Input: part model. Units: mm. Frame: model coordinates. A direction names the side the tool comes from. Give positions to 0.01 mm unless a question says otherwise; leave off trailing zeros. Loops run counter-clockwise (first coordinate to the right, second up) from the corner with the lowest first, then second, coordinate; pieces in that order, holes last.
from build123d import *

# Parameters (mm, degrees)
SKETCH1_W                               = 80
SKETCH1_H                               = 80
SKETCH1_R                               = 2.55
SKETCH1_R_2                             = 2.05
BOSS_EXTRUDE1_DEPTH                     = 7
CBORE_FOR_5_64_EJECTOR_PIN1_D           = 1.984375
CBORE_FOR_5_64_EJECTOR_PIN1_CBORE_D     = 5.953125
CBORE_FOR_5_64_EJECTOR_PIN1_CBORE_DEPTH = 2.175


with BuildPart() as part:
    # Sketch1 → Boss-Extrude1 (new body)
    with BuildSketch(Plane(origin=(0, 0, 0), x_dir=(1, 0, 0), z_dir=(0, 1, 0))):
        with Locations((0, 18)):
            Rectangle(SKETCH1_W, SKETCH1_H)
        with Locations((-30, 15)):
            Circle(SKETCH1_R, mode=Mode.SUBTRACT)
        with Locations((30, 15)):
            Circle(SKETCH1_R, mode=Mode.SUBTRACT)
        with Locations((30, -15)):
            Circle(SKETCH1_R, mode=Mode.SUBTRACT)
        with Locations((-30, -15)):
            Circle(SKETCH1_R, mode=Mode.SUBTRACT)
        with Locations((-26.5, 53)):
            Circle(SKETCH1_R_2, mode=Mode.SUBTRACT)
        with Locations((26.5, 53)):
            Circle(SKETCH1_R_2, mode=Mode.SUBTRACT)
        with Locations((26.5, 33)):
            Circle(SKETCH1_R_2, mode=Mode.SUBTRACT)
        with Locations((-26.5, 33)):
            Circle(SKETCH1_R_2, mode=Mode.SUBTRACT)
    extrude(amount=BOSS_EXTRUDE1_DEPTH)

    # CBORE for 5/64 Ejector Pin1 (through all)
    with Locations(Plane(origin=(0, 0, 0), x_dir=(-1, 0, 0), z_dir=(0, -1, 0))):
        with Locations((26.5, 33), (-26.5, 33), (26.5, 53), (-26.5, 53)):
            CounterBoreHole(CBORE_FOR_5_64_EJECTOR_PIN1_D / 2, CBORE_FOR_5_64_EJECTOR_PIN1_CBORE_D / 2, CBORE_FOR_5_64_EJECTOR_PIN1_CBORE_DEPTH)


solid = part.part
(1) Pin query (flat end, axial travel): pin 1 Ø1.8 at (x, z) = (25.5, -54) entering from -Y (3 decimals). Return the tip coordinate at first contact, or that it passes through.
Values follow:
pin 1: stops at y = 2.175
(2) Cut plane B-B (z = -53). Return the cut outline in (x, y) (3 decimals), and give its area (3 significant figures).
Values follow:
outline: (-40, 0) - (-29.477, 0) - (-29.477, 2.175) - (-28.55, 2.175) - (-28.55, 7) - (-40, 7) - close; (-24.45, 2.175) - (-23.523, 2.175) - (-23.523, 0) - (23.523, 0) - (23.523, 2.175) - (24.45, 2.175) - (24.45, 7) - (-24.45, 7) - close; (28.55, 2.175) - (29.477, 2.175) - (29.477, 0) - (40, 0) - (40, 7) - (28.55, 7) - close
area: 495 mm2
(3) Ray query, probe 1 along Z at (x, y) = (-26.5, 0.6); probe 2 along X at (y, z) = (1.3, -33); probe 3 along X at (y, z) = (4.3, -53). Return the intervals inside material, ascending.
Values follow:
probe 1: z = -58 to -55.98, -50.02 to -35.98, -30.02 to 22
probe 2: x = -40 to -29.48, -23.52 to 23.52, 29.48 to 40
probe 3: x = -40 to -28.55, -24.45 to 24.45, 28.55 to 40
(4) Mould query, pull axis Z, two halves, no side actions, for faces 1 (the flat face through (-40, 3, -17)), 2 (the flat face through (-24, 2.175, -32)), 3 (the flat face through (-1, 3, 22)). Classes: +Z half, -Z half, draft (parallel to the pull), parting line (faces both ways), or undercut.
Values follow:
face 1: draft
face 2: undercut
face 3: +Z half
(5) Reachability of faces 4 (the flat face through (29, 2.175, -32)), 5 (the cylindrical face through (-32.548, 3.451, 14.888)) from +Z, -Z, +X, -X, +Y, -Y: full face, straight path, thin tool, end or side. Return the list, or none.
Values follow:
face 4: -Y
face 5: +Y, -Y
(6) Cut plane D-D (z = -15). Return the cut outline in (x, y), and give its area (3 significant figures).
Values follow:
outline: (-40, 0) - (-32.55, 0) - (-32.55, 7) - (-40, 7) - close; (-27.45, 0) - (27.45, 0) - (27.45, 7) - (-27.45, 7) - close; (32.55, 0) - (40, 0) - (40, 7) - (32.55, 7) - close
area: 489 mm2
(7) Cut plane C-C (y = 6). Count the separate pieces of the cut face and the enclosed holes in it, and give its area (3 significant figures).
Values follow:
separate pieces: 1
enclosed holes: 8
area: 6,270 mm2
(8) Cut plane A-A (x = 26.5). Return the cut outline in (y, z) (3 decimals), and give its area (3 significant figures).
Values follow:
outline: (0, -58) - (7, -58) - (7, -55.05) - (2.175, -55.05) - (2.175, -55.977) - (0, -55.977) - close; (0, -50.023) - (2.175, -50.023) - (2.175, -50.95) - (7, -50.95) - (7, -35.05) - (2.175, -35.05) - (2.175, -35.977) - (0, -35.977) - close; (0, -30.023) - (2.175, -30.023) - (2.175, -30.95) - (7, -30.95) - (7, 22) - (0, 22) - close
area: 495 mm2
